```python
from build123d import *

# Parameters (mm, degrees)
SKETCH1_R           = 22.5
SKETCH1_R_2         = 3.5
BOSS_EXTRUDE1_DEPTH = 10


with BuildPart() as part:
    # Sketch1 → Boss-Extrude1 (new body)
    with BuildSketch(Plane.XY):
        with BuildLine():
            Line((46.8, 19.758542456), (46.8, -19.758542456))
            ThreePointArc((46.8, -19.758542456), (0, -50.8), (-46.8, -19.758542456))
            Line((-46.8, -19.758542456), (-46.8, 19.758542456))
            ThreePointArc((-46.8, 19.758542456), (0, 50.8), (46.8, 19.758542456))
        make_face()
        Circle(SKETCH1_R, mode=Mode.SUBTRACT)
        with Locations((0, 28.867513459)):
            Circle(SKETCH1_R_2, mode=Mode.SUBTRACT)
        with Locations((25, -14.43375673)):
            Circle(SKETCH1_R_2, mode=Mode.SUBTRACT)
        with Locations((-25, -14.43375673)):
            Circle(SKETCH1_R_2, mode=Mode.SUBTRACT)
    extrude(amount=BOSS_EXTRUDE1_DEPTH)

    # Sketch4 → M4x0.7 Tapped Hole1 (revolve, cut)
    with BuildSketch(Plane(origin=(46.8, 0, 5), x_dir=(0, 0, -1), z_dir=(0, 1, 0))):
        Polygon((0, 0), (0, 15.991420021), (1.65, 15), (1.65, 0), align=None)
    m4x0_7_tapped_hole1 = revolve(axis=Axis((53.15, 0, 5), (-1, 0, 0)), mode=Mode.SUBTRACT)

    # Mirror1: M4x0.7 Tapped Hole1 across plane
    add(m4x0_7_tapped_hole1.mirror(Plane(origin=(0, 0, 0), x_dir=(0, 0, 1), z_dir=(1, 0, 0))), mode=Mode.SUBTRACT)


solid = part.part
```
Geometry check sheet. Reference: the model listing, model coordinates, mm. A direction names the side the tool comes from. Round coordinates to 2 decimals unless told otherwise and drop trailing zeros. Order: outer loops, then holes, each group sorted by start corner. A loop starts at its lowest first (then second) coordinate and runs counter-clockwise, first axis right, second up. Notation, with made-up numbers: M -25,88.25 L 6,88.25 A7 cw 6,95.25 Z; hole C 54,-17 d3. An arc over 180 degrees is marked long. Answer as CSV lines item,"result".
1) Sectioned sample at B-B on y = -13. Record the cut outline in (x, z), and give its area (3 significant figures).
Entries:
outline,"M -46.8,0 L -28.19,0 L -28.19,10 L -46.8,10 Z; M -21.81,0 L -18.36,0 L -18.36,10 L -21.81,10 Z; M 18.36,0 L 21.81,0 L 21.81,10 L 18.36,10 Z; M 28.19,0 L 46.8,0 L 46.8,10 L 28.19,10 Z"
area,"441 mm2"
2) Sectioned sample at A-A on x = 0. Record the cut outline in (y, z), and give its area (3 significant figures).
Entries:
outline,"M -50.8,0 L -22.5,0 L -22.5,10 L -50.8,10 Z; M 22.5,0 L 25.37,0 L 25.37,10 L 22.5,10 Z; M 32.37,0 L 50.8,0 L 50.8,10 L 32.37,10 Z"
area,"496 mm2"
3) Thickness scan on probe 1 along Y at (x, z) = (0, 3); probe 2 along Z at (x, y) = (39, 0); probe 3 along Y at (x, z) = (-43.25, 5). Record the ranges inside material, lowest first. Write a range as [from, to].
Entries:
probe 1,"[-50.8, -22.5], [22.5, 25.37], [32.37, 50.8]"
probe 2,"[0, 3.35], [6.65, 10]"
probe 3,"[-26.65, -1.65], [1.65, 26.65]"
4) Tool access check on faces 1 (the face through (10.382, -19.961, 4.93)), 2 (the face through (-39.4, -0.07, 6.65)), 3 (the face through (39.4, -0.07, 6.65)). Record the directions out of +Z, -Z, +X, -X, +Y, -Y that give a thin tool (end or side, any length) a straight path to the whole face; none if there is none.
Entries:
face 1,"+Z, -Z"
face 2,"-X"
face 3,"+X"
5) Gauge pin test, flat ends, axial feed: pin 1 Ø1.5 at (y, z) = (33.5, 8) entering from +X; pin 2 Ø2.5 at (y, z) = (0, 5) entering from -X; pin 3 Ø2 at (x, z) = (27, 5) entering from +Y. Record the tip position at first contact, or that the pin passes through.
Entries:
pin 1,"x = 38.83"
pin 2,"x = -31.56"
pin 3,"y = 43.64"
6) Mould release check, pull along X, two halves, no side actions. Record for faces 4 (the face through (-21.662, -13.382, 4.93)), 5 (the face through (-0.833, 50.793, 4.93)), 6 (the face through (28.338, -13.382, 4.93)), 7 (the face through (30.981, -0.013, 5.286)): +X half, -X half, draft (parallel to the pull), parting line (faces both ways), or undercut.
Entries:
face 4,"undercut"
face 5,"parting line"
face 6,"undercut"
face 7,"+X half"
7) Sectioned sample at D-D on y = 4. Record the cut outline in (x, z).
Entries:
outline,"M -46.8,0 L -22.14,0 L -22.14,10 L -46.8,10 Z; M 22.14,0 L 46.8,0 L 46.8,10 L 22.14,10 Z"
8) Sectioned sample at C-C on x = 25. Record the cut outline in (y, z).
Entries:
outline,"M -44.22,0 L -17.93,0 L -17.93,10 L -44.22,10 Z; M -10.93,0 L 44.22,0 L 44.22,10 L -10.93,10 Z"
